```python
from build123d import *

# Parameters (mm, degrees)
SKETCH2_W             = 6.5
SKETCH2_H             = 6.5
RAILS_DEPTH           = 340.5
RAILS_2_DEPTH         = 340.5
SKETCH3_W             = 6.5
SKETCH3_H             = 87
FRONT_STRUT_DEPTH     = 1.5875
SKETCH4_W             = 6.5
SKETCH4_H             = 87
FRONT_MID_STRUT_DEPTH = 0.79375
SKETCH5_W             = 6.5
SKETCH5_H             = 87
BACK_MID_STRUT_DEPTH  = 0.79375
SKETCH6_W             = 6.5
SKETCH6_H             = 87
BACK_STRUT_DEPTH      = 1.5875
SKETCH7_W             = 4.9125
SKETCH7_H             = 87
X_SIDE_FLANGES_DEPTH  = 1.5875
SKETCH8_W             = 107.618749964
SKETCH8_H             = 4.9125
SKETCH8_W_2           = 105.912500092
FRAME_INSERTS_DEPTH   = 4.9125
SKETCH9_R             = 1.190625
Z_SCREWHOLES_DEPTH    = 349.70940624
SKETCH10_R            = 1.190625
X_SCREWHOLES_DEPTH    = 355.940135798


with BuildPart() as part:
    # Sketch2 → rails (new body)
    with BuildSketch(Plane.XY):
        with Locations((3.25, 3.25)):
            Rectangle(SKETCH2_W, SKETCH2_H)
    extrude(amount=-RAILS_DEPTH)



with BuildPart() as body_2:
    # Sketch2 → rails 2 (new body)
    with BuildSketch(Plane.XY):
        with Locations((3.25, 96.75)):
            Rectangle(SKETCH2_W, SKETCH2_H)
    extrude(amount=-RAILS_2_DEPTH)


with BuildPart() as part_1:
    add(part.part)

    add(body_2.part)  # front strut merges body 2
    # Sketch3 → front strut (add)
    with BuildSketch(Plane.XY.offset(-6.5)):
        with Locations((3.25, 50)):
            Rectangle(SKETCH3_W, SKETCH3_H)
    extrude(amount=-FRONT_STRUT_DEPTH)

    # Sketch4 → front mid strut (add, symmetric)
    with BuildSketch(Plane.XY.offset(-116.499999964)):
        with Locations((3.25, 50)):
            Rectangle(SKETCH4_W, SKETCH4_H)
    extrude(amount=FRONT_MID_STRUT_DEPTH, both=True)

    # Sketch5 → back mid strut (add, symmetric)
    with BuildSketch(Plane.XY.offset(-224.000000056)):
        with Locations((3.25, 50)):
            Rectangle(SKETCH5_W, SKETCH5_H)
    extrude(amount=BACK_MID_STRUT_DEPTH, both=True)

    # Sketch6 → back strut (add)
    with BuildSketch(Plane.XY.offset(-334.00000002)):
        with Locations((3.25, 50)):
            Rectangle(SKETCH6_W, SKETCH6_H)
    extrude(amount=BACK_STRUT_DEPTH)

    # Sketch7 → x side flanges (add)
    with BuildSketch(Plane(origin=(0, 0, 0), x_dir=(0, 0, -1), z_dir=(1, 0, 0))):
        with Locations((10.54375, 50)):
            Rectangle(SKETCH7_W, SKETCH7_H)
        with Locations((113.249999964, 50)):
            Rectangle(SKETCH7_W, SKETCH7_H)
        with Locations((119.749999964, 50)):
            Rectangle(SKETCH7_W, SKETCH7_H)
        with Locations((220.750000056, 50)):
            Rectangle(SKETCH7_W, SKETCH7_H)
        with Locations((227.250000056, 50)):
            Rectangle(SKETCH7_W, SKETCH7_H)
        with Locations((329.95625002, 50)):
            Rectangle(SKETCH7_W, SKETCH7_H)
    extrude(amount=X_SIDE_FLANGES_DEPTH)

    # Sketch8 → frame inserts (cut)
    with BuildSketch(Plane(origin=(6.5, 0, 0), x_dir=(0, 0, -1), z_dir=(1, 0, 0))):
        with Locations((61.896874982, 4.04375)):
            Rectangle(SKETCH8_W, SKETCH8_H)
        with Locations((61.896874982, 95.95625)):
            Rectangle(SKETCH8_W, SKETCH8_H)
        with Locations((170.25000001, 95.95625)):
            Rectangle(SKETCH8_W_2, SKETCH8_H)
        with Locations((170.25000001, 4.04375)):
            Rectangle(SKETCH8_W_2, SKETCH8_H)
        with Locations((278.603125038, 4.04375)):
            Rectangle(SKETCH8_W, SKETCH8_H)
        with Locations((278.603125038, 95.95625)):
            Rectangle(SKETCH8_W, SKETCH8_H)
    extrude(amount=-FRAME_INSERTS_DEPTH, mode=Mode.SUBTRACT)

    # Sketch9 → z screwholes (cut, through all)
    with BuildSketch(Plane.XY.offset(-6.5)):
        with Locations((4.11875, 88.1)):
            Circle(SKETCH9_R)
        with Locations((4.11875, 50)):
            Circle(SKETCH9_R)
        with Locations((4.11875, 11.9)):
            Circle(SKETCH9_R)
    extrude(amount=-Z_SCREWHOLES_DEPTH, mode=Mode.SUBTRACT)

    # Sketch10 → x screwholes (cut, through all)
    with BuildSketch(Plane(origin=(0, 0, 0), x_dir=(0, 0, -1), z_dir=(1, 0, 0))):
        with Locations(Location((10.61875, 95.88125, 0), (0, 0, 180))):
            Circle(SKETCH10_R)
        with Locations(Location((113.174999964, 95.88125, 0), (0, 0, 180))):
            Circle(SKETCH10_R)
        with Locations(Location((61.896874982, 95.88125, 0), (0, 0, 180))):
            Circle(SKETCH10_R)
        with Locations(Location((119.824999964, 95.88125, 0), (0, 0, 180))):
            Circle(SKETCH10_R)
        with Locations(Location((157.924999964, 95.88125, 0), (0, 0, 180))):
            Circle(SKETCH10_R)
        with Locations(Location((10.61875, 69.05, 0), (0, 0, 180))):
            Circle(SKETCH10_R)
        with Locations(Location((113.174999964, 69.05, 0), (0, 0, 180))):
            Circle(SKETCH10_R)
        with Locations(Location((119.824999964, 69.05, 0), (0, 0, 180))):
            Circle(SKETCH10_R)
        with Locations(Location((220.675000056, 69.05, 0), (0, 0, 180))):
            Circle(SKETCH10_R)
        with Locations(Location((227.325000056, 69.05, 0), (0, 0, 180))):
            Circle(SKETCH10_R)
        with Locations(Location((329.88125002, 69.05, 0), (0, 0, 180))):
            Circle(SKETCH10_R)
        with Locations(Location((182.575000056, 95.88125, 0), (0, 0, 180))):
            Circle(SKETCH10_R)
        with Locations(Location((220.675000056, 95.88125, 0), (0, 0, 180))):
            Circle(SKETCH10_R)
        with Locations(Location((278.603125038, 95.88125, 0), (0, 0, 180))):
            Circle(SKETCH10_R)
        with Locations(Location((227.325000056, 95.88125, 0), (0, 0, 180))):
            Circle(SKETCH10_R)
        with Locations(Location((329.88125002, 95.88125, 0), (0, 0, 180))):
            Circle(SKETCH10_R)
        with Locations(Location((329.88125002, 4.11875, 0), (0, 0, 180))):
            Circle(SKETCH10_R)
        with Locations(Location((227.325000056, 4.11875, 0), (0, 0, 180))):
            Circle(SKETCH10_R)
        with Locations(Location((278.603125038, 4.11875, 0), (0, 0, 180))):
            Circle(SKETCH10_R)
        with Locations(Location((220.675000056, 4.11875, 0), (0, 0, 180))):
            Circle(SKETCH10_R)
        with Locations(Location((182.575000056, 4.11875, 0), (0, 0, 180))):
            Circle(SKETCH10_R)
        with Locations(Location((329.88125002, 30.95, 0), (0, 0, 180))):
            Circle(SKETCH10_R)
        with Locations(Location((227.325000056, 30.95, 0), (0, 0, 180))):
            Circle(SKETCH10_R)
        with Locations(Location((220.675000056, 30.95, 0), (0, 0, 180))):
            Circle(SKETCH10_R)
        with Locations(Location((119.824999964, 30.95, 0), (0, 0, 180))):
            Circle(SKETCH10_R)
        with Locations(Location((113.174999964, 30.95, 0), (0, 0, 180))):
            Circle(SKETCH10_R)
        with Locations(Location((10.61875, 30.95, 0), (0, 0, 180))):
            Circle(SKETCH10_R)
        with Locations(Location((157.924999964, 4.11875, 0), (0, 0, 180))):
            Circle(SKETCH10_R)
        with Locations(Location((119.824999964, 4.11875, 0), (0, 0, 180))):
            Circle(SKETCH10_R)
        with Locations(Location((61.896874982, 4.11875, 0), (0, 0, 180))):
            Circle(SKETCH10_R)
        with Locations(Location((113.174999964, 4.11875, 0), (0, 0, 180))):
            Circle(SKETCH10_R)
        with Locations(Location((10.61875, 4.11875, 0), (0, 0, 180))):
            Circle(SKETCH10_R)
    extrude(amount=X_SCREWHOLES_DEPTH, mode=Mode.SUBTRACT)


solid = part_1.part
```
The model under review builds one solid part; all positions refer to its coordinate system, in mm. A direction names the side the tool comes from. Round coordinates to 2 decimals unless told otherwise and drop trailing zeros. Loops run counter-clockwise (first coordinate to the right, second up) from the corner with the lowest first, then second, coordinate; pieces in that order, holes last. Notation, with made-up numbers: (14, 48) - (49, 48) arc R25 ccw to (49, 64) - close; hole circle Ø7 at (25, 23). An arc over 180 degrees is marked (long way). Use a Markdown table: item, result. Add a question column.
Q1. For probe 1 along Z at (x, y) = (2, 53); probe 2 along Z at (x, y) = (5.75, 95.5); probe 3 along Y at (x, z) = (1.5, -278.5), list the stretches that pass through material, from the lowest coordinate up.
Q2. Add section B-B (x = 4). State how many separate pieces and enclosed holes the cut face has, plus the area to 3 significant figures.
Q3. Add section A-A (z = -145.5). State the section outline as (x, y) points, plus the area to 3 significant figures.
Q4. Insertion check: pin 1 Ø1.5 at (x, y) = (3, 69) entering from +Z; pin 2 Ø3 at (x, y) = (5, 78.5) entering from -Z; pin 3 Ø2 at (x, y) = (4.12, 50) entering from +Z; pin 4 Ø2.5 at (y, z) = (4.12, -157.92) entering from +X. Each pin has a flat end and moves straight along its axis. Give the tip position at first contact, or say it passes through.
Q5. The part is to be moulded in two halves that separate along Y. For faces 1 (the face through (3, 100, -168)), 2 (the face through (2, 51, -334)), 3 (the face through (0, 47, -220)), say which applies: pulls with the +Y half, pulls with the -Y half, needs draft (parallel to the pull), parting line crosses it, or undercut.
Q6. Machinability: for faces 4 (the face through (3, 6.5, -337)), 5 (the face through (3, 6.5, -3)), 6 (the face through (1.588, 97, -274)), 7 (the face through (6.5, 50, -333)), which of the approach directions +Z, -Z, +X, -X, +Y, -Y give a long, thin tool a straight path to every point of the face, cutting with its end or side? Answer none if there is none.
Worked answers:
| question | item | result |
|---|---|---|
| 1 | probe 1 | -334 to -332.41, -224.79 to -223.21, -117.29 to -115.71, -8.09 to -6.5 |
| 1 | probe 2 | -340.5 to -332.41, -224.79 to -223.21, -117.29 to -115.71, -8.09 to 0 |
| 1 | probe 3 | 0 to 2.93, 5.3 to 6.5, 93.5 to 94.7, 97.07 to 100 |
| 2 | separate pieces | 10 |
| 2 | enclosed holes | 0 |
| 2 | area | 1,780 mm² |
| 3 | outline | (0, 0) - (6.5, 0) - (6.5, 1.59) - (1.59, 1.59) - (1.59, 6.5) - (0, 6.5) - close; (0, 93.5) - (1.59, 93.5) - (1.59, 98.41) - (6.5, 98.41) - (6.5, 100) - (0, 100) - close |
| 3 | area | 36.2 mm² |
| 4 | pin 1 | z = -6.5 |
| 4 | pin 2 | z = -334 |
| 4 | pin 3 | through |
| 4 | pin 4 | x = 1.59 |
| 5 | face 1 | pulls with the +Y half |
| 5 | face 2 | undercut |
| 5 | face 3 | needs draft |
| 6 | face 4 | -Z, +X, -X |
| 6 | face 5 | +Z, +X, -X |
| 6 | face 6 | +X |
| 6 | face 7 | +Z, -Z, +X, +Y, -Y |
